Could you check a few things on this model? Use its own coordinates, in mm. A direction names the side the tool comes from. Round coordinates to 2 decimals unless told otherwise and drop trailing zeros. Loops run counter-clockwise (first coordinate to the right, second up) from the corner with the lowest first, then second, coordinate; pieces in that order, holes last. Notation, with made-up numbers: M 4,-19 L 59,-19 A29 ccw 59,15 Z; hole C 6,83.25 d4. An arc over 180 degrees is marked long. Return JSON: item names as keys, results as strings. Group by question number.
```python
from build123d import *

# Parameters (mm, degrees)
SKIZZE1_R                       = 4
SKIZZE1_R_2                     = 1.6
AUFSATZ_LINEAR_AUSTRAGEN1_DEPTH = 27
SKIZZE2_OUTSIDE_W               = 15.854
SKIZZE2_OUTSIDE_H               = 15.854
SKIZZE2_OUTSIDE_R               = 2.7425
SCHNITT_LINEAR_AUSTRAGEN1_DEPTH = 3
FASE1_SIZE                      = 0.4


with BuildPart() as part:
    # Skizze1 → Aufsatz-Linear austragen1 (new body)
    with BuildSketch(Plane(origin=(0, 0, 0), x_dir=(0, 0, -1), z_dir=(1, 0, 0))):
        Circle(SKIZZE1_R)
        Circle(SKIZZE1_R_2, mode=Mode.SUBTRACT)
    extrude(amount=AUFSATZ_LINEAR_AUSTRAGEN1_DEPTH)

    # Skizze2 outside → Schnitt-Linear austragen1 (cut)
    with BuildSketch(Plane(origin=(27, 0, 0), x_dir=(0, 0, -1), z_dir=(1, 0, 0))):
        Rectangle(SKIZZE2_OUTSIDE_W, SKIZZE2_OUTSIDE_H)
        Circle(SKIZZE2_OUTSIDE_R, mode=Mode.SUBTRACT)
    extrude(amount=-SCHNITT_LINEAR_AUSTRAGEN1_DEPTH, mode=Mode.SUBTRACT)

    # Fase1
    fase1_edges = [part.edges().sort_by_distance(p)[0] for p in [
        (0, 0, 1.6),
        (27, 0, 1.6),
    ]]
    chamfer(fase1_edges, length=FASE1_SIZE)


solid = part.part
```
1. If we section it at A-A, the plane y = 0: Please give me the cut outline in (x, z), then the cut area to 3 significant figures.
2. I'm going to push flat-ended pins straight in: pin 1 Ø3 at (x, z) = (3.5, 3) entering from -Y; pin 2 Ø3 at (x, y) = (14.5, -2.5) entering from +Z; pin 3 Ø1 at (x, z) = (17.5, -0.5) entering from -Y. Where does each tip first touch, or does it pass through?
3. We'd pull the mould along Y, two halves only. Please class faces 1 (the face through (11.832, -3.905, 0.867)), 2 (the face through (24, 1, -3)), 3 (the face through (13.32, -0.97, 1.27)): +Y half, -Y half, draft (parallel to the pull), parting line (faces both ways), or undercut.
4. If we section it at D-D, the plane y = -2.25: Please give me the cut outline in (x, z), then the cut area to 3 significant figures.
5. I need wall thicknesses on probe 1 along Y at (x, z) = (11, 0); probe 2 along Z at (x, y) = (25.5, 0.5); probe 3 along Y at (x, z) = (8.5, -1). Which ranges of each line are inside material? Lowest first, please.
6. On a 3-axis mill with a long thin cutter (end or side, diameter ignored), from which of +Z, -Z, +X, -X, +Y, -Y can I reach the whole of each face in a straight line? I mean faces 4 (the face through (25.52, -2.68, 0.59)), 5 (the face through (0, -1, 2)). Say none if no direction works.
7. If we section it at C-C, the plane x = 3: Please give me the cut outline in (y, z), then the cut area to 3 significant figures.
Geometry results:
{
 "1": {"outline": "M 0,-4 L 24,-4 L 24,-2.74 L 27,-2.74 L 27,-2 L 26.6,-1.6 L 0.4,-1.6 L 0,-2 Z; M 0,2 L 0.4,1.6 L 26.6,1.6 L 27,2 L 27,2.74 L 24,2.74 L 24,4 L 0,4 Z", "area": "122 mm^2"},
 "2": {"pin 1": "y = -3.71", "pin 2": "z = 3.87", "pin 3": "y = -4"},
 "3": {"face 1": "parting line", "face 2": "draft", "face 3": "undercut"},
 "4": {"outline": "M 0,-3.31 L 24,-3.31 L 24,-1.57 L 27,-1.57 L 27,1.57 L 24,1.57 L 24,3.31 L 0,3.31 Z", "area": "168 mm^2"},
 "5": {"probe 1": "-4 to -1.6, 1.6 to 4", "probe 2": "-2.7 to -1.52, 1.52 to 2.7", "probe 3": "-3.87 to -1.25, 1.25 to 3.87"},
 "6": {"face 4": "+X", "face 5": "+Z, -Z, -X, +Y, -Y"},
 "7": {"outline": "C 0,0 d8; hole C 0,0 d3.2", "area": "42.2 mm^2"}
}
